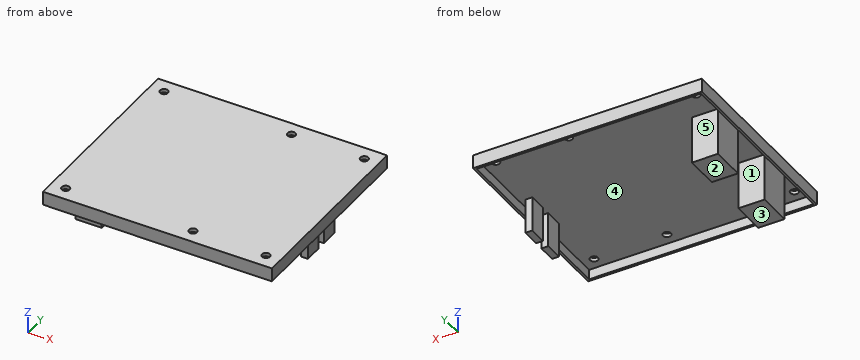
from build123d import *

# Parameters (mm, degrees)
SKETCH031_W             = 98.6
SKETCH031_H             = 84.6
PAD021_DEPTH            = 1.6
SKETCH032_W             = 100.6
SKETCH032_H             = 86.6
SKETCH032_W_2           = 98.6
SKETCH032_H_2           = 84.6
PAD022_DEPTH            = 6
SKETCH034_W             = 11.5
SKETCH034_H             = 15
PAD023_DEPTH            = 22.5
SKETCH035_W             = 3
SKETCH035_H             = 8
PAD024_DEPTH            = 17
SKETCH033_R             = 1.75
POCKET010_DEPTH         = 5
BODY007_PLACEMENT_ANGLE = 180


with BuildPart() as part:
    # Sketch031 → Pad021 (new body)
    with BuildSketch(Plane.XY):
        Rectangle(SKETCH031_W, SKETCH031_H)
    extrude(amount=PAD021_DEPTH)

    # Sketch032 → Pad022 (join)
    with BuildSketch(Plane.XY):
        Rectangle(SKETCH032_W, SKETCH032_H)
        Rectangle(SKETCH032_W_2, SKETCH032_H_2, mode=Mode.SUBTRACT)
    extrude(amount=PAD022_DEPTH)

    # Sketch034 → Pad023 (join)
    with BuildSketch(Plane.XY):
        with Locations((-40.95, 17.5)):
            Rectangle(SKETCH034_W, SKETCH034_H)
        with Locations((-40.95, -17.5)):
            Rectangle(SKETCH034_W, SKETCH034_H)
    extrude(amount=PAD023_DEPTH)

    # Sketch035 → Pad024 (join)
    with BuildSketch(Plane.XY):
        with Locations((45.2, 6)):
            Rectangle(SKETCH035_W, SKETCH035_H)
        with Locations((45.2, -6)):
            Rectangle(SKETCH035_W, SKETCH035_H)
    extrude(amount=PAD024_DEPTH)

    # Sketch033 → Pocket010 (cut)
    with BuildSketch(Plane.XY):
        with Locations((-44, 37)):
            Circle(SKETCH033_R)
        with Locations((12, 37)):
            Circle(SKETCH033_R)
        with Locations((44, 37)):
            Circle(SKETCH033_R)
        with Locations((44, -37)):
            Circle(SKETCH033_R)
        with Locations((12, -37)):
            Circle(SKETCH033_R)
        with Locations((-44, -37)):
            Circle(SKETCH033_R)
    extrude(amount=POCKET010_DEPTH, mode=Mode.SUBTRACT)


with BuildPart() as part_1:
    # Body007 placement: moved
    add(part.part.moved(Location((0, 0, 49.5))).rotate(Axis((0, 0, 49.5), (1, 0, 0)), BODY007_PLACEMENT_ANGLE))


solid = part_1.part
Work out the finished part from the listing and answer in its coordinate system (mm). Face numbers are marked on the shaded views. A direction names the side the tool comes from. Coordinates: 2 decimals unless noted, no trailing zeros. Loops run counter-clockwise (first coordinate to the right, second up) from the corner with the lowest first, then second, coordinate; pieces in that order, holes last. Notation, with made-up numbers: (-31.75, 65.5) -> (6.25, 65.5) arc R19 ccw to (6.25, 97.5) -> close; hole circle Ø9 at (72.25, 87.5). An arc over 180 degrees is marked (long way). Write each question's results on one line, items separated by ' | '. Start each with the question number.
1) Find section C-C on z = 29.5. Determine the outline of the cut face in (x, y), then the cut area to 3 significant figures.
2) Find section A-A on x = -44. Determine the outline of the cut face in (y, z), then the cut area to 3 significant figures.
3) The mould has two halves that part along Y. Classify the marked faces 3, 4 and 5: pulls with the +Y half, pulls with the -Y half, needs draft (parallel to the pull), parting line crosses it, or undercut.
4) Find section B-B on y = 37. Determine the outline of the cut face in (x, z), then the cut area to 3 significant figures.
5) For the marked faces 1 and 2, determine the directions among +Z, -Z, +X, -X, +Y, -Y from which every point of the face is accessible in a straight line to the end or side of a thin tool.
6) Flat-ended cylindrical pins translate along their axes: P1, Ø2, axis at x = 12, y = 37, coming from the +Z side; P2, Ø7.5, axis at y = -14.5, z = 37, coming from the -X side; P3, Ø3.5, axis at x = -42.5, z = 32.5, coming from the +Y side; P4, Ø2, axis at x = 16, y = 3.5, coming from the -Z side. Find the tip coordinate at first contact, or state that the pin passes through.
7) Consider line 1 along X through (y, z) = (37, 48.4); line 2 along Y through (x, z) = (44, 49); line 3 along X through (y, z) = (6, 44). Determine where each line is inside the solid, lowest interval first.
8) Find section D-D on y = -32. Determine the outline of the cut face in (x, z), then the cut area to 3 significant figures.
Response values:
1) outline: (-46.7, -25) -> (-35.2, -25) -> (-35.2, -10) -> (-46.7, -10) -> close; (-46.7, 10) -> (-35.2, 10) -> (-35.2, 25) -> (-46.7, 25) -> close | area: 345 mm^2
2) outline: (-43.3, 43.5) -> (-42.3, 43.5) -> (-42.3, 47.9) -> (-38.75, 47.9) -> (-38.75, 49.5) -> (-43.3, 49.5) -> close; (-35.25, 47.9) -> (-25, 47.9) -> (-25, 27) -> (-10, 27) -> (-10, 47.9) -> (10, 47.9) -> (10, 27) -> (25, 27) -> (25, 47.9) -> (35.25, 47.9) -> (35.25, 49.5) -> (-35.25, 49.5) -> close; (38.75, 47.9) -> (42.3, 47.9) -> (42.3, 43.5) -> (43.3, 43.5) -> (43.3, 49.5) -> (38.75, 49.5) -> close | area: 763 mm^2
3) face 3: needs draft | face 4: undercut | face 5: undercut
4) outline: (-50.3, 43.5) -> (-49.3, 43.5) -> (-49.3, 47.9) -> (-45.75, 47.9) -> (-45.75, 49.5) -> (-50.3, 49.5) -> close; (-42.25, 47.9) -> (10.25, 47.9) -> (10.25, 49.5) -> (-42.25, 49.5) -> close; (13.75, 47.9) -> (42.25, 47.9) -> (42.25, 49.5) -> (13.75, 49.5) -> close; (45.75, 47.9) -> (49.3, 47.9) -> (49.3, 43.5) -> (50.3, 43.5) -> (50.3, 49.5) -> (45.75, 49.5) -> close | area: 153 mm^2
5) face 1: -Z | face 2: -Z, +X, -X, +Y, -Y
6) P1: passes through | P2: stops at x = -46.7 | P3: stops at y = 25 | P4: stops at z = 47.9
7) line 1: x = -50.3 to -45.75, -42.25 to 10.25, 13.75 to 42.25, 45.75 to 50.3 | line 2: y = -43.3 to -38.75, -35.25 to 35.25, 38.75 to 43.3 | line 3: x = -50.3 to -49.3, 43.7 to 46.7, 49.3 to 50.3
8) outline: (-50.3, 43.5) -> (-49.3, 43.5) -> (-49.3, 47.9) -> (49.3, 47.9) -> (49.3, 43.5) -> (50.3, 43.5) -> (50.3, 49.5) -> (-50.3, 49.5) -> close | area: 170 mm^2
